Here's how the part is built. I have some questions about the finished solid (model axes, mm). Face numbers are marked on the shaded views. A direction names the side the tool comes from. Round coordinates to 2 decimals unless told otherwise and drop trailing zeros. Order: outer loops, then holes, each group sorted by start corner. A loop starts at its lowest first (then second) coordinate and runs counter-clockwise, first axis right, second up.
```python
from build123d import *

# Parameters (mm, degrees)
SKETCH1_W           = 20
SKETCH1_H           = 20
BOSS_EXTRUDE1_DEPTH = 20
CUT_EXTRUDE2_DEPTH  = 28
CUT_EXTRUDE3_DEPTH  = 8.55
CUT_EXTRUDE4_DEPTH  = 17.1
CUT_EXTRUDE5_DEPTH  = 17.1


with BuildPart() as part:
    # Sketch1 → Boss-Extrude1 (new body)
    with BuildSketch(Plane.XY):
        Rectangle(SKETCH1_W, SKETCH1_H)
    extrude(amount=BOSS_EXTRUDE1_DEPTH)

    # Sketch3 → Cut-Extrude2 (cut)
    with BuildSketch(Plane(origin=(10, 0, 0), x_dir=(0, 0, -1), z_dir=(1, 0, 0))):
        Polygon((-3.2, 10), (-20, -6.8), (-20, 10), align=None)
    extrude(amount=-CUT_EXTRUDE2_DEPTH, mode=Mode.SUBTRACT)

    # Sketch6 → Cut-Extrude3 (cut, symmetric)
    with BuildSketch(Plane.ZY):
        Polygon((3.2, 10), (3.2, -6.8), (20, -6.8), align=None)
    extrude(amount=CUT_EXTRUDE3_DEPTH, both=True, mode=Mode.SUBTRACT)

    # Sketch7 → Cut-Extrude4 (cut)
    with BuildSketch(Plane.XY.offset(3.2)):
        with BuildLine():
            Line((-2.25, 0), (-2.25, 4))
            ThreePointArc((-2.25, 4), (0, 6.25), (2.25, 4))
            Line((2.25, 4), (2.25, 0))
            ThreePointArc((2.25, 0), (0, -2.25), (-2.25, 0))
        make_face()
    extrude(amount=-CUT_EXTRUDE4_DEPTH, mode=Mode.SUBTRACT)

    # Sketch9 → Cut-Extrude5 (cut)
    with BuildSketch(Plane(origin=(0, -6.8, 0), x_dir=(1, 0, 0), z_dir=(0, 1, 0))):
        with BuildLine():
            Line((2.25, -10), (2.25, -14))
            ThreePointArc((2.25, -14), (0, -16.25), (-2.25, -14))
            Line((-2.25, -14), (-2.25, -10))
            ThreePointArc((-2.25, -10), (0, -7.75), (2.25, -10))
        make_face()
    extrude(amount=-CUT_EXTRUDE5_DEPTH, mode=Mode.SUBTRACT)


solid = part.part
```
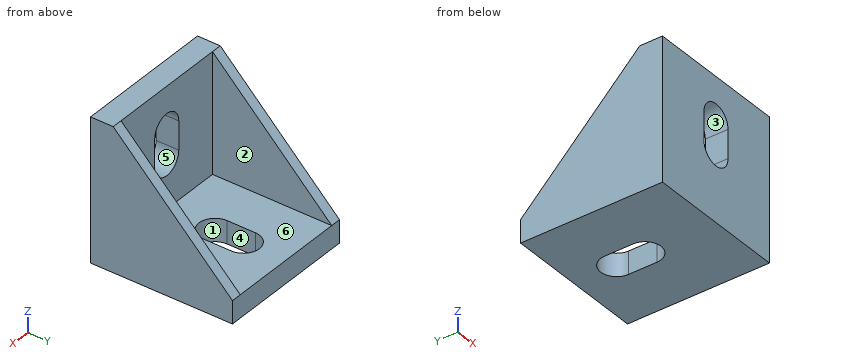
1. I need wall thicknesses on probe 1 along X at (y, z) = (2.75, 7); probe 2 along X at (y, z) = (1, 2.5); probe 3 along Y at (x, z) = (1, 4.25). Which ranges of each line are inside material? Lowest first, please.
Evaluation:
probe 1: x = -10 to -8.55, 8.55 to 10
probe 2: x = -10 to -2.25, 2.25 to 10
probe 3: y = -10 to -6.8
2. If we section it at B-B, the plane z = 13.5: Write out the boundary of the cut face in (x, y).
Evaluation:
outline: (-10, -10) - (-2.25, -10) - (-2.25, -6.8) - (-8.55, -6.8) - (-8.55, -0.3) - (-10, -0.3) - close; (2.25, -10) - (10, -10) - (10, -0.3) - (8.55, -0.3) - (8.55, -6.8) - (2.25, -6.8) - close
3. If we section it at C-C, the plane x = 0: Write out the boundary of the cut face in (y, z).
Evaluation:
outline: (-10, 0) - (-2.25, 0) - (-2.25, 3.2) - (-6.8, 3.2) - (-6.8, 7.75) - (-10, 7.75) - close; (-10, 16.25) - (-6.8, 16.25) - (-6.8, 20) - (-10, 20) - close; (6.25, 0) - (10, 0) - (10, 3.2) - (6.25, 3.2) - close
4. On a 3-axis mill with a long thin cutter (end or side, diameter ignored), from which of +Z, -Z, +X, -X, +Y, -Y can I reach the whole of each face in a straight line? I mean the marked faces 1, 2 and 3. Say none if no direction works.
Evaluation:
face 1: +Z, -Z
face 2: +Z, +Y
face 3: +Y, -Y
5. If we mould it in two halves opening along Z, with no side actions, what happens to the marked faces 4, 5 and 6? For each: released by +Z, released by -Z, zero draft, split by the parting line, or undercut.
Evaluation:
face 4: zero draft
face 5: undercut
face 6: released by +Z
6. If we section it at D-D, the plane x = -7.5: Write out the boundary of the cut face in (y, z).
Evaluation:
outline: (-10, 0) - (10, 0) - (10, 3.2) - (-6.8, 3.2) - (-6.8, 20) - (-10, 20) - close
7. I'm going to push flat-ended pins straight in: P1, Ø4, axis at x = 8, z = 17.5, coming from the +Y side; P2, Ø1, axis at x = 0, z = 16, coming from the +Y side; P3, Ø1.5, axis at x = 1.5, y = 5.5, coming from the +Z side. Where does each tip first touch, or does it pass through?
Evaluation:
P1: stops at y = -2.38
P2: stops at y = -6.8
P3: stops at z = 3.2
8. If we section it at A-A, the plane y = 3: Write out the boundary of the cut face in (x, z).
Evaluation:
outline: (-10, 0) - (-2.25, 0) - (-2.25, 3.2) - (-8.55, 3.2) - (-8.55, 10.2) - (-10, 10.2) - close; (2.25, 0) - (10, 0) - (10, 10.2) - (8.55, 10.2) - (8.55, 3.2) - (2.25, 3.2) - close
